Check sheet for the modelled part. Datum: model origin and axes. Units: mm. A direction names the side the tool comes from. Round coordinates to 2 decimals unless told otherwise and drop trailing zeros. Loops run counter-clockwise (first coordinate to the right, second up) from the corner with the lowest first, then second, coordinate; pieces in that order, holes last. Notation, with made-up numbers: (-36.75, 77.25) - (-21.75, 77.25) arc R20 cw to (-21.75, 84.25) - close; hole circle Ø4 at (72, 65.5). An arc over 180 degrees is marked (long way). Put each result on its own line as item: value.
```python
from build123d import *

# Parameters (mm, degrees)
BOSS_EXTRUDE1_DEPTH = 20
FILLET1_R           = 5


with BuildPart() as part:
    # Sketch1 → Boss-Extrude1 (new body)
    with BuildSketch(Plane(origin=(0, 0, 0), x_dir=(1, 0, 0), z_dir=(0, 1, 0))):
        Polygon((-75, 15), (-75, -15), (-63.3, -15), (-63.3, 8), (-47.8, 8), (-47.8, -15), (-32.8, -15), (-32.8, 8), (-17.3, 8), (-17.3, -15), (17.3, -15), (17.3, 8), (32.8, 8), (32.8, -15), (47.8, -15), (47.8, 8), (63.3, 8), (63.3, -15), (75, -15), (75, 15), align=None)
    extrude(amount=BOSS_EXTRUDE1_DEPTH)

    # Fillet1
    fillet1_edges = [part.edges().sort_by_distance(p)[0] for p in [
        (0, 20, -15),
    ]]
    fillet(fillet1_edges, radius=FILLET1_R)


solid = part.part
```
Item 1: Section check A-A on z = -3.25. Enter the section's corners in (x, y), then the cut area to 3 significant figures.
Filled sheet:
outline: (-75, 0) - (-63.3, 0) - (-63.3, 20) - (-75, 20) - close; (-47.8, 0) - (-32.8, 0) - (-32.8, 20) - (-47.8, 20) - close; (-17.3, 0) - (17.3, 0) - (17.3, 20) - (-17.3, 20) - close; (32.8, 0) - (47.8, 0) - (47.8, 20) - (32.8, 20) - close; (63.3, 0) - (75, 0) - (75, 20) - (63.3, 20) - close
area: 1,760 mm²
Item 2: Section check D-D on z = -13. Enter the section's corners in (x, y).
Filled sheet:
outline: (-75, 0) - (75, 0) - (75, 19) - (-75, 19) - close
Item 3: Tool access check on faces 1 (the flat face through (75, 10, 0)), 2 (the flat face through (25, 10, -8)). Record the directions out of +Z, -Z, +X, -X, +Y, -Y that give a thin tool (end or side, any length) a straight path to the whole face; none if there is none.
Filled sheet:
face 1: +Z, -Z, +X, +Y, -Y
face 2: +Z, +Y, -Y
Item 4: Go/stop test with a flat-tipped pin: pin 1 (7.5 mm diameter, centred on x = -23.5, y = 14.5, fed in from +Z). Record where the tip stops, or that it passes through.
Filled sheet:
pin 1: z = -8
Item 5: Section check B-B on y = 4. Enter the section's corners in (x, z), then the cut area to 3 significant figures.
Filled sheet:
outline: (-75, -15) - (75, -15) - (75, 15) - (63.3, 15) - (63.3, -8) - (47.8, -8) - (47.8, 15) - (32.8, 15) - (32.8, -8) - (17.3, -8) - (17.3, 15) - (-17.3, 15) - (-17.3, -8) - (-32.8, -8) - (-32.8, 15) - (-47.8, 15) - (-47.8, -8) - (-63.3, -8) - (-63.3, 15) - (-75, 15) - close
area: 3,070 mm²
Item 6: Section check C-C on x = -51.5. Enter the section's corners in (y, z).
Filled sheet:
outline: (0, -15) - (15, -15) arc R5 ccw to (20, -10) - (20, -8) - (0, -8) - close
Item 7: Thickness scan on line 1 (X direction, y = 7, z = 8.75); line 2 (Z direction, x = 27, y = 4.25); line 3 (Z direction, x = -57.5, y = 17.25). Record the ranges inside material, lowest first. Write a range as from..to.
Filled sheet:
line 1: -75..-63.3, -47.8..-32.8, -17.3..17.3, 32.8..47.8, 63.3..75
line 2: -15..-8
line 3: -14.47..-8
